Here's how the part is built. I have some questions about the finished solid (model axes, mm). Face numbers are marked on the shaded views. A direction names the side the tool comes from. Coordinates: 2 decimals unless noted, no trailing zeros. Loops run counter-clockwise (first coordinate to the right, second up) from the corner with the lowest first, then second, coordinate; pieces in that order, holes last. Notation, with made-up numbers: (-27, -38.75) -> (-23, -38.75) arc R29 cw to (-23, -3.75) -> close; hole circle Ø4 at (42.5, -23). An arc over 180 degrees is marked (long way). Use CSV: the item, a comma, the result in double quotes. Start each with the question number.
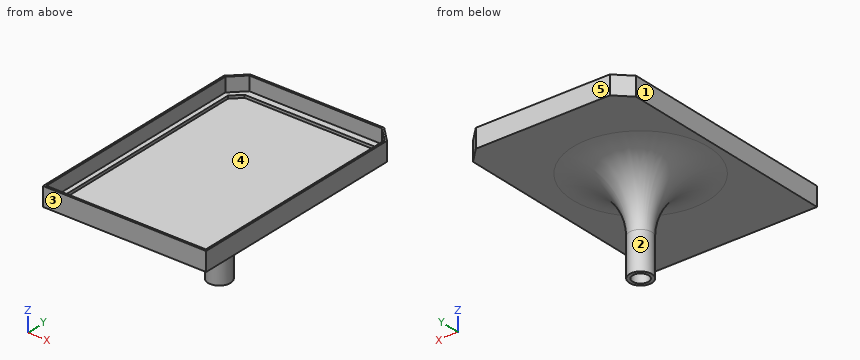
from build123d import *

# Parameters (mm, degrees)
BOSS_EXTRUDE1_DEPTH = 1.5
BOSS_EXTRUDE2_DEPTH = 9
BOSS_EXTRUDE3_DEPTH = 1
SKETCH4_R           = 6
SKETCH4_R_2         = 4.25
BOSS_EXTRUDE4_DEPTH = 50
SKETCH5_R           = 6
SKETCH5_R_2         = 4.25
BOSS_EXTRUDE5_DEPTH = 20
FILLET1_R           = 30


with BuildPart() as part:
    # Sketch1 → Boss-Extrude1 (new body)
    with BuildSketch(Plane(origin=(0, 0, 0), x_dir=(0, 1, 0), z_dir=(0, 0, 1))):
        Polygon((-62.5, -42.5), (-62.5, 42.5), (55.428932188, 42.5), (62.5, 35.428932188), (62.5, -35.428932188), (55.428932188, -42.5), align=None)
        Polygon((54.050252532, 40), (59, 35.050252532), (59, -35.050252532), (54.050252532, -40), (-59, -40), (-59, 40), align=None, mode=Mode.SUBTRACT)
    extrude(amount=BOSS_EXTRUDE1_DEPTH)

    # Sketch2 → Boss-Extrude2 (add)
    with BuildSketch(Plane(origin=(0, 0, 0), x_dir=(0, 1, 0), z_dir=(0, 0, 1))):
        Polygon((-63.5, 43.5), (-63.5, -43.5), (55.721825407, -43.5), (63.5, -35.721825407), (63.5, 35.721825407), (55.721825407, 43.5), align=None)
        Polygon((-62.5, -42.5), (55.428932188, -42.5), (62.5, -35.428932188), (62.5, 35.428932188), (55.428932188, 42.5), (-62.5, 42.5), align=None, mode=Mode.SUBTRACT)
    extrude(amount=BOSS_EXTRUDE2_DEPTH)

    # Sketch3 → Boss-Extrude3 (add)
    with BuildSketch(Plane(origin=(0, 0, 0), x_dir=(0, 1, 0), z_dir=(0, 0, 1))):
        Polygon((55.721825407, 43.5), (-63.5, 43.5), (-63.5, -43.5), (55.721825407, -43.5), (63.5, -35.721825407), (63.5, 35.721825407), align=None)
    extrude(amount=-BOSS_EXTRUDE3_DEPTH)

    # Sketch4 → Boss-Extrude4 (add)
    with BuildSketch(Plane(origin=(0, 0, -1), x_dir=(1, 0, 0), z_dir=(0, 0, -1))):
        with Locations((-4.3, -4.3)):
            Circle(SKETCH4_R)
        with Locations(Location((-4.3, -4.3, 0), (0, 0, 180))):
            Circle(SKETCH4_R_2, mode=Mode.SUBTRACT)
    extrude(amount=BOSS_EXTRUDE4_DEPTH)

    # Sketch5 → Boss-Extrude5 (add)
    with BuildSketch(Plane(origin=(0, 0, -1), x_dir=(1, 0, 0), z_dir=(0, 0, -1))):
        with Locations((-4.3, -4.3)):
            Circle(SKETCH5_R)
        with Locations(Location((-4.3, -4.3, 0), (0, 0, 180))):
            Circle(SKETCH5_R_2, mode=Mode.SUBTRACT)
    extrude(amount=BOSS_EXTRUDE5_DEPTH)

    # Fillet1
    fillet1_edges = [part.edges().sort_by_distance(p)[0] for p in [
        (-10.3, 4.3, -1),
    ]]
    fillet(fillet1_edges, radius=FILLET1_R)


solid = part.part
1) For P1, Ø1, axis at x = -2.5, y = 22.5, coming from the +Z side; P2, Ø12, axis at y = -5.5, z = -45, coming from the +X side, each with a flat end and sliding along its axis, tell me the tip position at first contact or that it passes through.
2) Which directions (+Z, -Z, +X, -X, +Y, -Y) give clear straight access to the entire face, cutting with the end or side of a thin tool? Please do the marked faces 1 and 2.
3) I want a section at A-A, the plane z = 3.5. Please give me the cut outline in (x, y).
4) Thinking about a two-plate mould opening in Y: for the marked faces 3, 4 and 5, which applies, pulls with the +Y half, pulls with the -Y half, needs draft (parallel to the pull), parting line crosses it, or undercut?
5) Please list where these lines run through material, in increasing order: L1, parallel to X at y = 19, z = 7; L2, parallel to Y at x = -4, z = -39; L3, parallel to X at y = 4, z = -38. Write a range as [from, to].
6) I want a section at C-C, the plane x = -4.3. Please give me the cut outline in (y, z).
7) I want a section at B-B, the plane y = 4.3. Please give me the cut outline in (x, z).
8) I want a section at D-D, the plane z = -46. Please give me the cut outline in (x, y).
Return value:
1,P1,"stops at z = 0"
1,P2,"stops at x = 0.34"
2,face 1,"+Z, -Z, -X, +Y, -Y"
2,face 2,"-Z"
3,outline,"(-43.5, -63.5) -> (43.5, -63.5) -> (43.5, 55.72) -> (35.72, 63.5) -> (-35.72, 63.5) -> (-43.5, 55.72) -> close; hole (-42.5, -62.5) -> (42.5, -62.5) -> (42.5, 55.43) -> (35.43, 62.5) -> (-35.43, 62.5) -> (-42.5, 55.43) -> close"
4,face 3,"pulls with the -Y half"
4,face 4,"undercut"
4,face 5,"pulls with the +Y half"
5,L1,"x = [-43.5, -42.5], [42.5, 43.5]"
5,L2,"y = [-1.69, 0.06], [8.54, 10.29]"
5,L3,"x = [-10.29, -8.54], [-0.06, 1.69]"
6,outline,"(-63.5, -1) -> (-31.7, -1) arc R30 cw to (-1.7, -31) -> (-1.7, -51) -> (0.05, -51) -> (0.05, -1) -> (8.55, -1) -> (8.55, -51) -> (10.3, -51) -> (10.3, -31) arc R30 cw to (40.3, -1) -> (63.5, -1) -> (63.5, 9) -> (62.5, 9) -> (62.5, 1.5) -> (59, 1.5) -> (59, 0) -> (-59, 0) -> (-59, 1.5) -> (-62.5, 1.5) -> (-62.5, 9) -> (-63.5, 9) -> close"
7,outline,"(-43.5, -1) -> (-40.3, -1) arc R30 cw to (-10.3, -31) -> (-10.3, -51) -> (-8.55, -51) -> (-8.55, -1) -> (-0.05, -1) -> (-0.05, -51) -> (1.7, -51) -> (1.7, -31) arc R30 cw to (31.7, -1) -> (43.5, -1) -> (43.5, 9) -> (42.5, 9) -> (42.5, 1.5) -> (40, 1.5) -> (40, 0) -> (-40, 0) -> (-40, 1.5) -> (-42.5, 1.5) -> (-42.5, 9) -> (-43.5, 9) -> close"
8,outline,"circle Ø12 at (-4.3, 4.3); hole circle Ø8.5 at (-4.3, 4.3)"
